Could you check a few things on this drawing? It's one solid part, dimensions in mm from its lowest x, y, z. A direction names the side the tool comes from. Give positions to 0.01 mm unless a question says otherwise; leave off trailing zeros. Write each loop counter-clockwise with the first axis right and the second up, starting at its lowest first coordinate (ties: lowest second). Pieces come first, ordered by that corner, then holes. Notation, with made-up numbers: (67, 56.5) -> (109, 56.5) arc R26 cw to (109, 71.5) -> close; hole circle Ø5 at (-38.75, 67). An arc over 180 degrees is marked (long way). Answer as CSV lines item,"result". Start each with the question number.
1. If we section it at C-C on y = 3: Write out the boundary of the cut face in (x, z), plus the area to 3 significant figures.
2. I need wall thicknesses on line 1 (Z direction, x = 7.9, y = 3.5); line 2 (Y direction, x = 1.5, z = 5.25); line 3 (Z direction, x = 7.25, y = 8.5). Which ranges of each line are inside material? Lowest first, please. Write a range as [from, to].
3. If we section it at A-A on x = 7.9: Write out the boundary of the cut face in (y, z).
4. I'm going to push flat-ended pins straight in: P1, Ø3, axis at x = 7.9, z = 7.9, coming from the -Y side; P2, Ø5, axis at x = 5, y = 5.5, coming from the +Z side; P3, Ø1.5, axis at x = 2, y = 4, coming from the -Z side; P4, Ø1.5, axis at y = 4, z = 4, coming from the -X side. Where does each tip first touch, or does it pass through?
5. If we section it at B-B on z = 7.9: Write out the boundary of the cut face in (x, y).
6. On a 3-axis mill with a long thin cutter (end or side, diameter ignored), from which of +Z, -Z, +X, -X, +Y, -Y can I reach the whole of each face in a straight line? I mean the marked faces 4 and 5. Say none if no direction works.
7. If we mould it in two halves opening along Z, with no side actions, what happens to the marked faces 1, 2 and 3? For each: pulls with the +Z half, pulls with the -Z half, needs draft (parallel to the pull), parting line crosses it, or undercut.
8. If we section it at D-D on x = 5.25: Write out the boundary of the cut face in (y, z), plus the area to 3 significant figures.
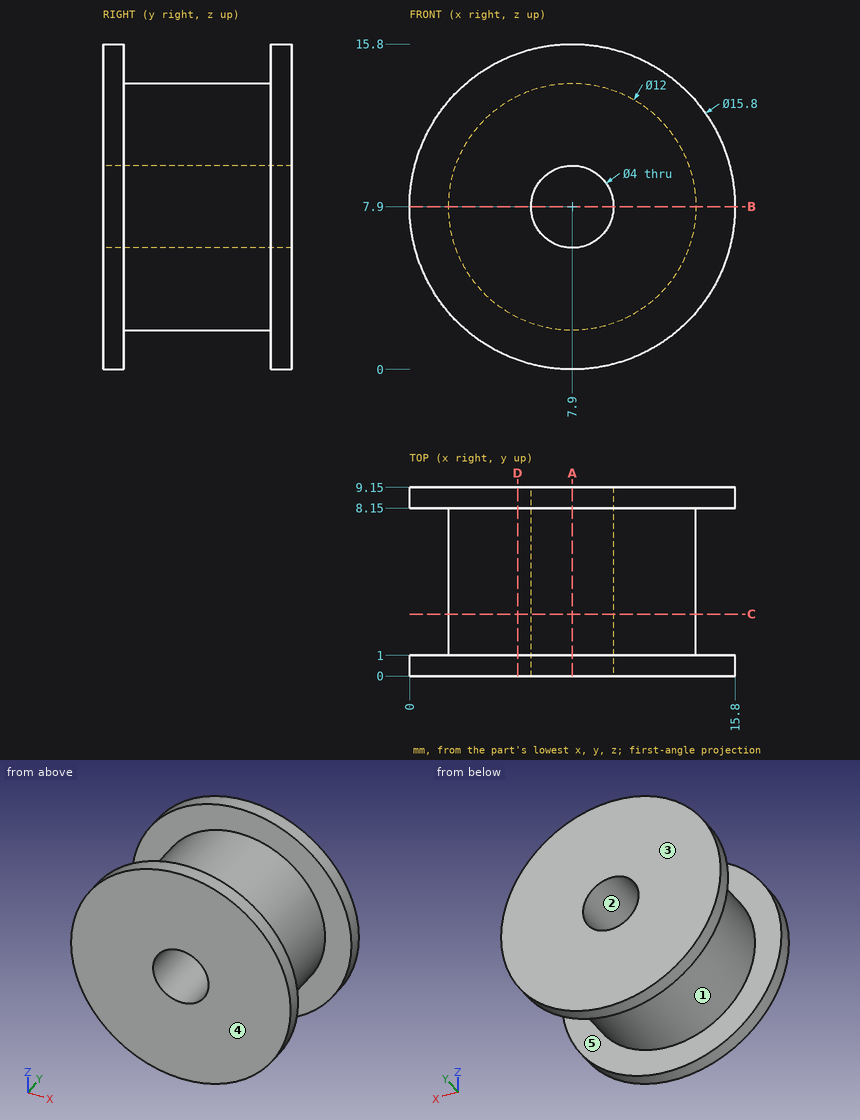
Computed values:
1,outline,"circle Ø12 at (7.9, 7.9); hole circle Ø4 at (7.9, 7.9)"
1,area,"101 mm2"
2,line 1,"z = [1.9, 5.9], [9.9, 13.9]"
2,line 2,"y = [0, 1], [8.15, 9.15]"
2,line 3,"z = [0.03, 6.01], [9.79, 15.77]"
3,outline,"(0, 0) -> (1, 0) -> (1, 1.9) -> (8.15, 1.9) -> (8.15, 0) -> (9.15, 0) -> (9.15, 5.9) -> (0, 5.9) -> close; (0, 9.9) -> (9.15, 9.9) -> (9.15, 15.8) -> (8.15, 15.8) -> (8.15, 13.9) -> (1, 13.9) -> (1, 15.8) -> (0, 15.8) -> close"
4,P1,"passes through"
4,P2,"stops at z = 13.89"
4,P3,"stops at z = 4.82"
4,P4,"stops at x = 2.79"
5,outline,"(0, 0) -> (5.9, 0) -> (5.9, 9.15) -> (0, 9.15) -> (0, 8.15) -> (1.9, 8.15) -> (1.9, 1) -> (0, 1) -> close; (9.9, 0) -> (15.8, 0) -> (15.8, 1) -> (13.9, 1) -> (13.9, 8.15) -> (15.8, 8.15) -> (15.8, 9.15) -> (9.9, 9.15) -> close"
6,face 4,"+Z, -Z, +X, -X, -Y"
6,face 5,"none"
7,face 1,"parting line crosses it"
7,face 2,"undercut"
7,face 3,"needs draft"
8,outline,"(0, 0.46) -> (1, 0.46) -> (1, 2.52) -> (8.15, 2.52) -> (8.15, 0.46) -> (9.15, 0.46) -> (9.15, 15.34) -> (8.15, 15.34) -> (8.15, 13.28) -> (1, 13.28) -> (1, 15.34) -> (0, 15.34) -> close"
8,area,"107 mm2"
